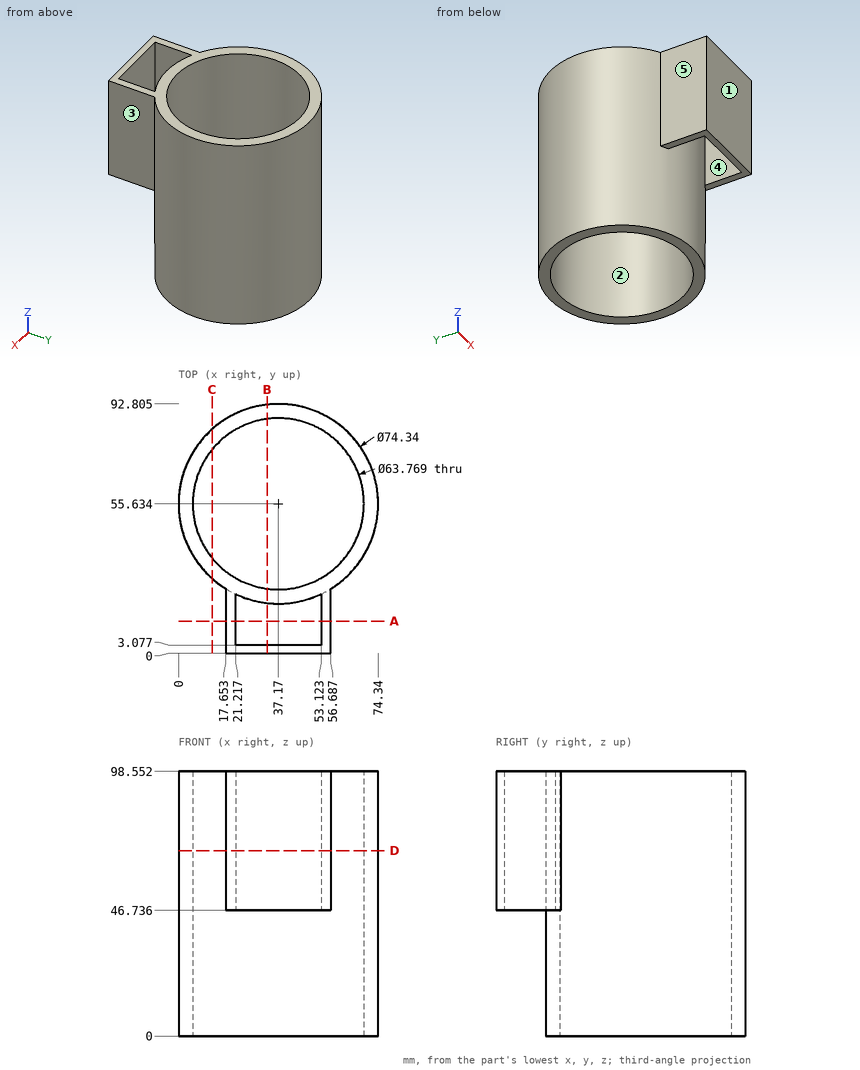
Design review of the part shown in the three views and the two pictorial views. Dimensions are in mm from the part's minimum x, y and z. A direction names the side the tool comes from. Coordinates: 2 decimals unless noted, no trailing zeros. Write each loop counter-clockwise with the first axis right and the second up, starting at its lowest first coordinate (ties: lowest second). Pieces come first, ordered by that corner, then holes.
1) We need section B-B on x = 33. State the section outline as (y, z) points (1 decimal), then the cut area to 3 significant figures.
2) To check wall thickness, follow probe 1 along X at (y, z) = (13, 57); probe 2 along Y at (x, z) = (44.5, 75.5) (1 decimal); probe 3 along X at (y, z) = (56.5, 56.5). State the ranges of each line that lie inside material, in increasing order.
3) Machinability: for the marked faces 4 and 5, which of the approach directions +Z, -Z, +X, -X, +Y, -Y give a long, thin tool a straight path to every point of the face, cutting with its end or side? Answer none if there is none.
4) We need section C-C on x = 12.5. State the section outline as (y, z) points (1 decimal), then the cut area to 3 significant figures.
5) We need section A-A on y = 12. State the section outline as (x, z) points.
6) The part is to be moulded in two halves that separate along X. For the marked faces 1, 2 and 3, say which applies: pulls with the +X half, pulls with the -X half, needs draft (parallel to the pull), parting line crosses it, or undercut.
7) Clearance check with flat-ended pins moving along their axes: pin 1 Ø2 at (x, z) = (12.5, 31.5) entering from +Y (1 decimal); pin 2 Ø10 at (x, y) = (16, 15.5) entering from -Z; pin 3 Ø8 at (y, z) = (48.5, 78) entering from -X; pin 4 Ø10 at (x, y) = (35.5, 33.5) entering from -Z. State where each tip first meets the part, or that it passes through.
8) We need section D-D on z = 69. State the section outline as (x, y) points (1 decimal), then the cut area to 3 significant figures.
Answer list:
1. outline: (0, 46.7) - (3.1, 46.7) - (3.1, 98.6) - (0, 98.6) - close; (18.7, 0) - (24, 0) - (24, 98.6) - (18.7, 98.6) - close; (87.2, 0) - (92.6, 0) - (92.6, 98.6) - (87.2, 98.6) - close
1. area: 1,210 mm2
2. probe 1: x = 17.65 to 21.22, 53.12 to 56.69
2. probe 2: y = 0 to 3.1, 19.2 to 24.6, 86.7 to 92.1
2. probe 3: x = 0.01 to 5.3, 69.04 to 74.33
3. face 4: +Z, -Z
3. face 5: +Z, -Z, -X, -Y
4. outline: (27.8, 0) - (35.4, 0) - (35.4, 98.6) - (27.8, 98.6) - close; (75.8, 0) - (83.4, 0) - (83.4, 98.6) - (75.8, 98.6) - close
4. area: 1,500 mm2
5. outline: (17.65, 46.74) - (21.22, 46.74) - (21.22, 98.55) - (17.65, 98.55) - close; (53.12, 46.74) - (56.69, 46.74) - (56.69, 98.55) - (53.12, 98.55) - close
6. face 1: needs draft
6. face 2: undercut
6. face 3: pulls with the +X half
7. pin 1: stops at y = 84.3
7. pin 2: stops at z = 46.74
7. pin 3: stops at x = 0.13
7. pin 4: passes through
8. outline: (17.7, 0) - (56.7, 0) - (56.7, 24) arc R37.2 ccw (long way) to (17.7, 24) - close; hole circle Ø63.8 at (37.2, 55.6); hole (21.2, 3.1) - (53.1, 3.1) - (53.1, 22.1) arc R37.2 cw to (21.2, 22.1) - close
8. area: 1,410 mm2
